from build123d import *

# Parameters (mm, degrees)
SKETCH15_R         = 5
BASE_EXTRUDE_DEPTH = 100
SKETCH24_OUTSIDE_W = 32.2
SKETCH24_OUTSIDE_H = 32.2
SKETCH24_OUTSIDE_R = 3.5
FRONT_CUT_DEPTH    = 10
FRONT_HOLE_D       = 3
FRONT_HOLE_DEPTH   = 10
FRONT_HOLE_TIP     = 0.901290929
CHAMFER1_SIZE      = 1
KEYWAY_CUT_START   = -25
KEYWAY_CUT_DEPTH   = 25
BACK_HOLE_D        = 4
BACK_HOLE_DEPTH    = 10
BACK_HOLE_TIP      = 1.201721238


with BuildPart() as part:
    # Sketch15 → Base Extrude (new body)
    with BuildSketch(Plane.XY):
        Circle(SKETCH15_R)
    extrude(amount=BASE_EXTRUDE_DEPTH)

    # Sketch24 outside → Front Cut (cut)
    with BuildSketch(Plane.XY.offset(100)):
        Rectangle(SKETCH24_OUTSIDE_W, SKETCH24_OUTSIDE_H)
        Circle(SKETCH24_OUTSIDE_R, mode=Mode.SUBTRACT)
    extrude(amount=-FRONT_CUT_DEPTH, mode=Mode.SUBTRACT)

    # Front Hole
    with Locations(Plane(origin=(0.062150556, -0.00731183, 100), x_dir=(1, 0, 0), z_dir=(0, 0, 1))):
        with Locations((0, 0)):
            Hole(FRONT_HOLE_D / 2, depth=FRONT_HOLE_DEPTH)
            with Locations((0, 0, -(FRONT_HOLE_DEPTH + FRONT_HOLE_TIP / 2))):  # 118° drill point
                Cone(0, FRONT_HOLE_D / 2, FRONT_HOLE_TIP, mode=Mode.SUBTRACT)

    # Chamfer1
    chamfer1_edges = [part.edges().sort_by_distance(p)[0] for p in [
        (-3.5, 0, 100),
    ]]
    chamfer(chamfer1_edges, length=CHAMFER1_SIZE)

    # Keyway → Keyway-Cut (cut)
    with BuildSketch(Plane.XY.offset(100).offset(KEYWAY_CUT_START)):
        with BuildLine():
            ThreePointArc((5, 0), (4.74341649, 1.58113883), (4, 3))
            Line((4, 3), (4, -3))
            ThreePointArc((4, -3), (4.74341649, -1.58113883), (5, 0))
        make_face()
    extrude(amount=KEYWAY_CUT_DEPTH, mode=Mode.SUBTRACT)

    # Back Hole
    with Locations(Plane(origin=(0, 0, 0), x_dir=(-1, 0, 0), z_dir=(0, 0, -1))):
        with Locations((0, 0)):
            Hole(BACK_HOLE_D / 2, depth=BACK_HOLE_DEPTH)
            with Locations((0, 0, -(BACK_HOLE_DEPTH + BACK_HOLE_TIP / 2))):  # 118° drill point
                Cone(0, BACK_HOLE_D / 2, BACK_HOLE_TIP, mode=Mode.SUBTRACT)


solid = part.part
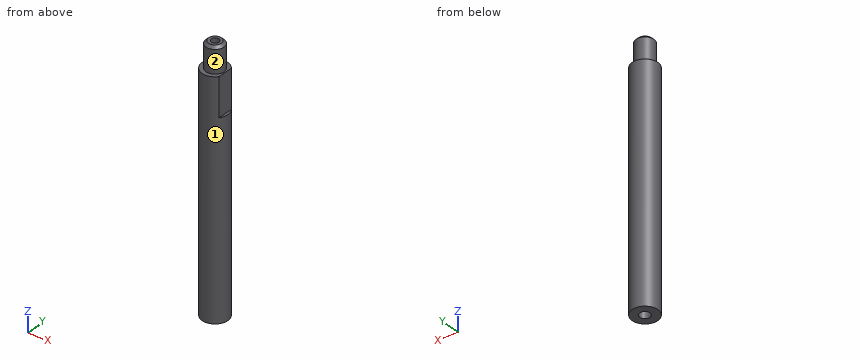
The model under review builds one solid part; all positions refer to its coordinate system, in mm. Face numbers are marked on the shaded views. A direction names the side the tool comes from. Round coordinates to 2 decimals unless told otherwise and drop trailing zeros. Write each loop counter-clockwise with the first axis right and the second up, starting at its lowest first coordinate (ties: lowest second). Pieces come first, ordered by that corner, then holes. Notation, with made-up numbers: M 9,42.25 L 22,42.25 A31 cw 22,73.25 Z; hole C 45.5,60.5 d2. An arc over 180 degrees is marked long. Use a Markdown table: item, result. Add a question column.
Q1. Machinability: for the marked faces 1 and 2, which of the approach directions +Z, -Z, +X, -X, +Y, -Y give a long, thin tool a straight path to every point of the face, cutting with its end or side? Answer none if there is none.
Q2. We need section A-A, the plane z = 64. State the section outline as (x, y) points.
Q3. We need section B-B, the plane z = 93. State the section outline as (x, y) points, plus the area to 3 significant figures.
Q4. Insertion check: pin 1 (1 mm diameter, centred on x = 3, z = 61, fed in from +Y); pin 2 (4.5 mm diameter, centred on x = 0, y = 0, fed in from -Z); pin 3 (1.1 mm diameter, centred on x = 4.5, y = 1, fed in from +Z); pin 4 (3.5 mm diameter, centred on x = 0.06, y = -0.01, fed in from -Z). Each pin has a flat end and moves straight along its axis. Give the tip position at first contact, or say it passes through.
Q5. To check wall thickness, follow line 1 (Y direction, x = -0.25, z = 4); line 2 (X direction, y = 0, z = 6.25); line 3 (X direction, y = 4, z = 60). State the ranges of each line that lie inside material, in increasing order.
Findings below:
| question | item | result |
|---|---|---|
| 1 | face 1 | +Z, -Z |
| 1 | face 2 | +Z |
| 2 | outline | C 0,0 d10 |
| 3 | outline | C 0,0 d7; hole C 0.06,-0.01 d3 |
| 3 | area | 31.4 mm² |
| 4 | pin 1 | stops at y = 4.33 |
| 4 | pin 2 | stops at z = 0 |
| 4 | pin 3 | stops at z = 90 |
| 4 | pin 4 | stops at z = 10.11 |
| 5 | line 1 | y = -4.99 to -1.98, 1.98 to 4.99 |
| 5 | line 2 | x = -5 to -2, 2 to 5 |
| 5 | line 3 | x = -3 to 3 |
